The listing builds one solid part. Answer for the finished solid, in the listing's coordinates (mm). Face numbers are marked on the shaded views. A direction names the side the tool comes from. Round coordinates to 2 decimals unless told otherwise and drop trailing zeros. Write each loop counter-clockwise with the first axis right and the second up, starting at its lowest first coordinate (ties: lowest second). Pieces come first, ordered by that corner, then holes.
(1) A cutting plane is placed at A-A, the plane z = 15. Give the vertices of the cut face in (x, y).
(2) Find the intervals of material crossed by probe 1 along Y at (x, z) = (17.5, 17); probe 2 along Z at (x, y) = (39.5, -45); probe 3 along Y at (x, z) = (1, 4), in increasing order.
(3) A cutting plane is placed at D-D, the plane z = 46. Give the vertices of the cut face in (x, y), and give its area (3 significant figures).
(4) Each of these flat-tipped pins is pushed along its axis until it touches: pin 1 Ø0.9 at (x, z) = (-42, 24) entering from -Y; pin 2 Ø6 at (x, z) = (-34.5, 20.5) entering from +Y; pin 3 Ø2 at (x, y) = (19, 14) entering from +Z. Where does it stop, or does it pass through?
(5) For the marked faces 5 and 6, determine the directions among +Z, -Z, +X, -X, +Y, -Y from which every point of the face is accessible in a straight line to the end or side of a thin tool.
(6) A cutting plane is placed at B-B, the plane x = -2.5. Give the vertices of the cut face in (y, z).
(7) A cutting plane is placed at C-C, the plane y = 17. Give the vertices of the cut face in (x, z).
(8) The mould has two halves that part along Z. Classify the marked faces 1, 2, 3 and 4: +Z half, -Z half, draft (parallel to the pull), parting line (faces both ways), or undercut.
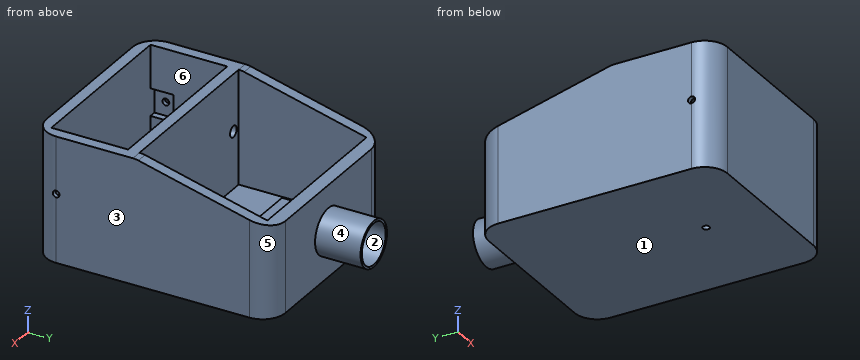
from build123d import *

# Parameters (mm, degrees)
SKETCH1_W               = 75
SKETCH1_H               = 95
BOSS_EXTRUDE4_DEPTH     = 50
BOSS_EXTRUDE5_START     = 5
BOSS_EXTRUDE5_DEPTH     = 5
CUT_EXTRUDE4_DEPTH      = 110.201648339
CUT_EXTRUDE4_DEPTH_BACK = 110.201648339
SKETCH7_R               = 1.5
SKETCH10_W              = 12
SKETCH10_H              = 10
CUT_EXTRUDE5_DEPTH      = 3
SKETCH11_W              = 12
SKETCH11_H              = 10
CUT_EXTRUDE6_DEPTH      = 3
CUT_EXTRUDE7_DEPTH      = 113.915898075
FILLET11_R              = 10
SKETCH13_W              = 50
SKETCH13_H              = 5
BOSS_EXTRUDE7_DEPTH     = 75
SKETCH17_R              = 1.5
CUT_EXTRUDE9_DEPTH      = 5
SKETCH18_W              = 21
SKETCH18_H              = 5
BOSS_EXTRUDE8_DEPTH     = 17
SKETCH21_R              = 2.5
CUT_EXTRUDE10_DEPTH     = 17
SKETCH22_R              = 10
SKETCH22_R_2            = 9
BOSS_EXTRUDE9_DEPTH     = 20
CUT_EXTRUDE11_START     = -5
SKETCH24_R              = 9
CUT_EXTRUDE11_DEPTH     = 5


with BuildPart() as part:
    # Sketch1 → Boss-Extrude4 (new body)
    with BuildSketch(Plane.XY):
        with BuildLine():
            Line((-35, -55), (30, -55))
            ThreePointArc((30, -55), (37.071067812, -52.071067812), (40, -45))
            Line((40, -45), (40, 40))
            ThreePointArc((40, 40), (37.071067812, 47.071067812), (30, 50))
            Line((30, 50), (-35, 50))
            ThreePointArc((-35, 50), (-42.071067812, 47.071067812), (-45, 40))
            Line((-45, 40), (-45, -45))
            ThreePointArc((-45, -45), (-42.071067812, -52.071067812), (-35, -55))
        make_face()
        with Locations((-2.5, -2.5)):
            Rectangle(SKETCH1_W, SKETCH1_H, mode=Mode.SUBTRACT)
    extrude(amount=BOSS_EXTRUDE4_DEPTH)

    # Sketch5 → Boss-Extrude5 (add)
    with BuildSketch(Plane(origin=(0, 0, 0), x_dir=(-1, 0, 0), z_dir=(0, 0, -1)).offset(BOSS_EXTRUDE5_START)):
        with BuildLine():
            Line((-30, -55), (35, -55))
            ThreePointArc((35, -55), (42.071067812, -52.071067812), (45, -45))
            Line((45, -45), (45, 40))
            ThreePointArc((45, 40), (42.071067812, 47.071067812), (35, 50))
            Line((35, 50), (-30, 50))
            ThreePointArc((-30, 50), (-37.071067812, 47.071067812), (-40, 40))
            Line((-40, 40), (-40, -45))
            ThreePointArc((-40, -45), (-37.071067812, -52.071067812), (-30, -55))
        make_face()
    extrude(amount=-BOSS_EXTRUDE5_DEPTH)

    # Sketch7 → Cut-Extrude4 (cut, two sides: drawn at the far end of the back side and taken through both)
    with BuildSketch(Plane.ZY.offset(-35).offset(-CUT_EXTRUDE4_DEPTH_BACK)):
        with Locations(Location((25, -45, 0), (0, 0, 180))):
            Circle(SKETCH7_R)
    extrude(amount=CUT_EXTRUDE4_DEPTH + CUT_EXTRUDE4_DEPTH_BACK, mode=Mode.SUBTRACT)

    # Sketch10 → Cut-Extrude5 (cut)
    with BuildSketch(Plane.ZY.offset(-35)):
        with Locations((25, -45)):
            Rectangle(SKETCH10_W, SKETCH10_H)
    extrude(amount=-CUT_EXTRUDE5_DEPTH, mode=Mode.SUBTRACT)

    # Sketch11 → Cut-Extrude6 (cut)
    with BuildSketch(Plane(origin=(-40, 0, 0), x_dir=(0, 0, -1), z_dir=(1, 0, 0))):
        with Locations((-25, -45)):
            Rectangle(SKETCH11_W, SKETCH11_H)
    extrude(amount=-CUT_EXTRUDE6_DEPTH, mode=Mode.SUBTRACT)

    # Sketch12 → Cut-Extrude7 (cut, through all)
    with BuildSketch(Plane(origin=(40, 0, 0), x_dir=(0, 0, -1), z_dir=(1, 0, 0))):
        Polygon((-50, -10), (-35, 50), (-50, 50), align=None)
    extrude(amount=-CUT_EXTRUDE7_DEPTH, mode=Mode.SUBTRACT)

    # Fillet11
    fillet11_edges = [part.edges().sort_by_distance(p)[0] for p in [
        (-42.5, -10, 50),
        (37.5, -10, 50),
    ]]
    fillet(fillet11_edges, radius=FILLET11_R)

    # Sketch13 → Boss-Extrude7 (add)
    with BuildSketch(Plane(origin=(-40, 0, 0), x_dir=(0, 0, -1), z_dir=(1, 0, 0))):
        with Locations((-25, -13.731056256)):
            Rectangle(SKETCH13_W, SKETCH13_H)
    extrude(amount=BOSS_EXTRUDE7_DEPTH)

    # Sketch17 → Cut-Extrude9 (cut)
    with BuildSketch(Plane.XY):
        with Locations((-2.5, -26.731056256)):
            Circle(SKETCH17_R)
    extrude(amount=-CUT_EXTRUDE9_DEPTH, mode=Mode.SUBTRACT)

    # Sketch18 → Boss-Extrude8 (add)
    with BuildSketch(Plane.XY):
        with Locations((-2.5, 26.060865593)):
            Rectangle(SKETCH18_W, SKETCH18_H)
    extrude(amount=BOSS_EXTRUDE8_DEPTH)

    # Sketch21 → Cut-Extrude10 (cut)
    with BuildSketch(Plane(origin=(0, -11.231056256, 0), x_dir=(1, 0, 0), z_dir=(0, 1, 0))):
        with Locations(Location((-36, -24.990851146, 0), (0, 0, 270))):
            Circle(SKETCH21_R)
        with Locations(Location((31, -24.990851146, 0), (0, 0, 270))):
            Circle(SKETCH21_R)
    extrude(amount=-CUT_EXTRUDE10_DEPTH, mode=Mode.SUBTRACT)

    # Sketch22 → Boss-Extrude9 (add)
    with BuildSketch(Plane(origin=(0, 50, 0), x_dir=(1, 0, 0), z_dir=(0, 1, 0))):
        with Locations(Location((-2.5, -15, 0), (0, 0, 90))):
            Circle(SKETCH22_R)
        with Locations(Location((-2.5, -15, 0), (0, 0, 270))):
            Circle(SKETCH22_R_2, mode=Mode.SUBTRACT)
    extrude(amount=BOSS_EXTRUDE9_DEPTH)

    # Sketch24 → Cut-Extrude11 (cut)
    with BuildSketch(Plane(origin=(0, 50, 0), x_dir=(1, 0, 0), z_dir=(0, 1, 0)).offset(CUT_EXTRUDE11_START)):
        with Locations(Location((-2.5, -15, 0), (0, 0, 270))):
            Circle(SKETCH24_R)
    extrude(amount=CUT_EXTRUDE11_DEPTH, mode=Mode.SUBTRACT)


solid = part.part
Solutions:
1. outline: (-45, -45) arc R10 ccw to (-35, -55) - (30, -55) arc R10 ccw to (40, -45) - (40, 40) arc R10 ccw to (30, 50) - (7.5, 50) - (7.5, 70) - (6.5, 70) - (6.5, 45) - (35, 45) - (35, -11.23) - (-40, -11.23) - (-40, 45) - (-11.5, 45) - (-11.5, 70) - (-12.5, 70) - (-12.5, 50) - (-35, 50) arc R10 ccw to (-45, 40) - close; (-13, 23.56) - (8, 23.56) - (8, 28.56) - (-13, 28.56) - close; hole (-40, -50) - (35, -50) - (35, -16.23) - (-40, -16.23) - close
2. probe 1: y = -55 to -50, -16.23 to -11.23, 45 to 50
2. probe 2: z = -5 to 23.5, 26.5 to 50
2. probe 3: y = -55 to -50, -16.23 to -11.23, 23.56 to 28.56, 45 to 50
3. outline: (-45, -45) arc R10 ccw to (-35, -55) - (30, -55) arc R10 ccw to (40, -45) - (40, 6) - (35, 6) - (35, -11.23) - (-40, -11.23) - (-40, 6) - (-45, 6) - close; hole (-40, -50) - (35, -50) - (35, -16.23) - (-40, -16.23) - close
3. area: 1,320 mm2
4. pin 1: stops at y = -52.56
4. pin 2: stops at y = 50
4. pin 3: stops at z = 0
5. face 5: +Z, -Z, +X, +Y
5. face 6: +Z
6. outline: (-55, -5) - (-28.23, -5) - (-28.23, 0) - (-50, 0) - (-50, 50) - (-55, 50) - close; (-25.23, -5) - (50, -5) - (50, 5) - (70, 5) - (70, 6) - (45, 6) - (45, 0) - (28.56, 0) - (28.56, 17) - (23.56, 17) - (23.56, 0) - (-11.23, 0) - (-11.23, 50) - (-16.23, 50) - (-16.23, 0) - (-25.23, 0) - close; (45, 24) - (70, 24) - (70, 25) - (50, 25) - (50, 35) - (45, 36.25) - close
7. outline: (-45, -5) - (40, -5) - (40, 43.25) - (35, 43.25) - (35, 0) - (-40, 0) - (-40, 43.25) - (-45, 43.25) - close
8. face 1: -Z half
8. face 2: undercut
8. face 3: draft
8. face 4: parting line
